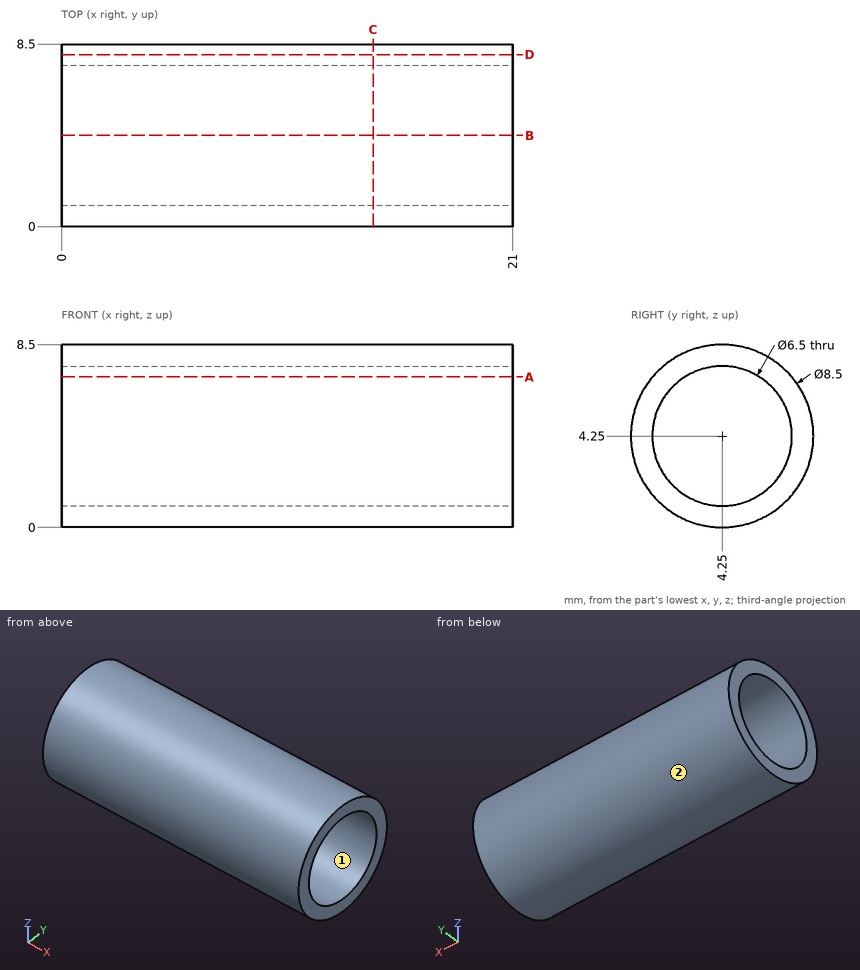
Design review of the part shown in the three views and the two pictorial views. Dimensions are in mm from the part's minimum x, y and z. Round coordinates to 2 decimals unless told otherwise and drop trailing zeros. Loops run counter-clockwise (first coordinate to the right, second up) from the corner with the lowest first, then second, coordinate; pieces in that order, holes last. Notation, with made-up numbers: (89, 21) -> (121, 21) arc R34 cw to (121, 51) -> close; hole circle Ø10 at (75, -14). An arc over 180 degrees is marked (long way). Answer as CSV lines item,"result".
1) Add section C-C on x = 14.5. Write out the cut boundary in (y, z), plus the area to 3 significant figures.
Geometry results:
outline,"circle Ø8.5 at (4.25, 4.25); hole circle Ø6.5 at (4.25, 4.25)"
area,"23.6 mm²"
2) Add section A-A on z = 7. Write out the cut boundary in (x, y), plus the area to 3 significant figures.
Geometry results:
outline,"(0, 1.01) -> (21, 1.01) -> (21, 2.52) -> (0, 2.52) -> close; (0, 5.98) -> (21, 5.98) -> (21, 7.49) -> (0, 7.49) -> close"
area,"63.3 mm²"
3) Add section D-D on y = 8. Write out the cut boundary in (x, z), plus the area to 3 significant figures.
Geometry results:
outline,"(0, 2.25) -> (21, 2.25) -> (21, 6.25) -> (0, 6.25) -> close"
area,"84.0 mm²"
4) Draft analysis for pull direction Y (two halves, no side actions). For the marked faces 1 and 2, state which applies: pulls with the +Y half, pulls with the -Y half, needs draft (parallel to the pull), parting line crosses it, or undercut.
Geometry results:
face 1,"undercut"
face 2,"parting line crosses it"
5) To check wall thickness, follow line 1 along Z through (x, y) = (5.5, 4.25); line 2 along Z through (x, y) = (2, 6.75). State the ranges of each line that lie inside material, in increasing order. Write a range as from..to.
Geometry results:
line 1,"z = 0..1, 7.5..8.5"
line 2,"z = 0.81..2.17, 6.33..7.69"
6) Add section B-B on y = 4.25. Write out the cut boundary in (x, z).
Geometry results:
outline,"(0, 0) -> (21, 0) -> (21, 1) -> (0, 1) -> close; (0, 7.5) -> (21, 7.5) -> (21, 8.5) -> (0, 8.5) -> close"
7) For P1, Ø2, axis at x = 5, y = 4.5, coming from the -Z side; P2, Ø1, axis at x = 9, z = 3, coming from the +Y side; P3, Ø5, axis at x = 7, z = 7.5, coming from the -Y side, all flat-tipped, find the tip position at first contact; note any pin that passes through.
Geometry results:
P1,"stops at z = 0"
P2,"stops at y = 8.43"
P3,"stops at y = 0.07"
